```python
from build123d import *

# Parameters (mm, degrees)
TD_SKETCH_R                             = 0.79248
TL_FEATURE_DEPTH                        = 21.0312
TDF_STD_SKETCH_W                        = 2.09296
TDF_STD_SKETCH_H                        = 2.09296
TDF_STD_FEATURE_DEPTH                   = 22.061040395
ISA_20_STD_FEATURE_DEPTH                = 22.061040395
ISA_20_STD_FEATURE_DEPTH_BACK           = 22.061040395
F_10BA_STD_FEATURE_DEPTH                = 22.061040395
F_10BA_STD_FEATURE_DEPTH_BACK           = 22.061040395
FRO_STD_FEATURE_DEPTH                   = 22.061040395
FRO_STD_FEATURE_DEPTH_BACK              = 22.061040395
C_STD_FEATURE_DEPTH                     = 22.061040395
C_STD_FEATURE_DEPTH_BACK                = 22.061040395
ERW_STD_FEATURE_DEPTH                   = 0.028575
H_STD_FEATURE_REACH                     = 22.881
H_STD_SKETCH_R                          = 0.01905
H_STD_SKETCH_3_R                        = 0.01905
FUNNEL_FINAL_DIAMETRE_STD_FEATURE_DEPTH = 2.499995
FUNNEL_FINAL_DIAMETRE_STD_FEATURE_DRAFT = -22.5
ROUND_BR_STD_FEATURE_START              = -1
ROUND_BR_STD_FEATURE_DEPTH              = 1.020088772


with BuildPart() as part:
    # TD_sketch → TL_feature (new body)
    with BuildSketch(Plane(origin=(0, 0, 0), x_dir=(1, 0, 0), z_dir=(0, 1, 0))):
        with Locations(Location((0, 0, 0), (0, 0, 270))):
            Circle(TD_SKETCH_R)
    extrude(amount=TL_FEATURE_DEPTH)

    # TDF_STD_sketch → TDF_STD_feature (cut, through all)
    with BuildSketch(Plane(origin=(0, 0, 0), x_dir=(1, 0, 0), z_dir=(0, 1, 0))):
        with Locations((-1.4224, 0)):
            Rectangle(TDF_STD_SKETCH_W, TDF_STD_SKETCH_H)
    extrude(amount=TDF_STD_FEATURE_DEPTH, mode=Mode.SUBTRACT)

    # ISA_20_STD_sketch → ISA_20_STD_feature (cut, two sides: drawn at the far end of the back side and taken through both)
    with BuildSketch(Plane(origin=(0, 0, 0), x_dir=(0, 0, -1), z_dir=(1, 0, 0)).offset(-ISA_20_STD_FEATURE_DEPTH_BACK)):
        Polygon((-12.952451681, 73.255332957), (-3.743927997, 21.0312), (-0.03556, 0), (0.03556, 0), (3.743927997, 21.0312), (12.952451681, 73.255332957), (12.952451681, -32.804215817), (-12.952451681, -32.804215817), align=None)
    extrude(amount=ISA_20_STD_FEATURE_DEPTH + ISA_20_STD_FEATURE_DEPTH_BACK, mode=Mode.SUBTRACT)

    # 10BA_STD_sketch → 10BA_STD_feature (cut, two sides: drawn at the far end of the back side and taken through both)
    with BuildSketch(Plane.XY.offset(-F_10BA_STD_FEATURE_DEPTH_BACK)):
        Polygon((-53.226091717, 0), (-0.37592, 0), (-0.28702, 0), (0.014453164, 0.053157853), (3.713447997, 21.0312), (12.890784005, 73.078458855), (91.272293615, 2.163710365), (25.155417893, -70.914748491), align=None)
    extrude(amount=F_10BA_STD_FEATURE_DEPTH + F_10BA_STD_FEATURE_DEPTH_BACK, mode=Mode.SUBTRACT)

    # FRO_STD_sketch → FRO_STD_feature (cut, two sides: drawn at the far end of the back side and taken through both)
    with BuildSketch(Plane.XY.offset(-FRO_STD_FEATURE_DEPTH_BACK)):
        with BuildLine():
            Line((-0.37592, 52.147609748), (-0.37592, 0.02286))
            ThreePointArc((-0.37592, 0.02286), (-0.369224461, 0.006695539), (-0.35306, 0))
            Line((-0.35306, 0), (51.771689748, 0))
            Line((51.771689748, 0), (-21.943838281, -73.715528029))
            Line((-21.943838281, -73.715528029), (-74.091448029, -21.567918281))
            Line((-74.091448029, -21.567918281), (-0.37592, 52.147609748))
        make_face()
    extrude(amount=FRO_STD_FEATURE_DEPTH + FRO_STD_FEATURE_DEPTH_BACK, mode=Mode.SUBTRACT)

    # C_STD_sketch → C_STD_feature (cut, two sides: drawn at the far end of the back side and taken through both)
    with BuildSketch(Plane(origin=(0, 0, 0), x_dir=(0, 0, -1), z_dir=(1, 0, 0)).offset(-C_STD_FEATURE_DEPTH_BACK)):
        with BuildLine():
            Line((-50.946547499, -11.043402092), (-0.035537314, 0))
            ThreePointArc((-0.035537314, 0), (0, 0.00381), (0.035537314, 0))
            Line((0.035537314, 0), (50.946547499, -11.043402092))
            Line((50.946547499, -11.043402092), (50.946547499, -115.233376423))
            Line((50.946547499, -115.233376423), (-50.946547499, -115.233376423))
            Line((-50.946547499, -115.233376423), (-50.946547499, -11.043402092))
        make_face()
    extrude(amount=C_STD_FEATURE_DEPTH + C_STD_FEATURE_DEPTH_BACK, mode=Mode.SUBTRACT)


with BuildPart() as body_2:
    # ERW_STD_sketch → ERW_STD_feature (new, symmetric)
    with BuildSketch(Plane.XY):
        Polygon((-0.127, 0.09652), (-0.127, 0), (-0.3175, 0), (-0.261774152, 0.09652), align=None)
    extrude(amount=ERW_STD_FEATURE_DEPTH, both=True)

    # H_STD_sketch → H_STD_feature (add, up to next)
    with BuildSketch(Plane(origin=(0.01693898, 0.179623209, 0), x_dir=(0, 0, -1), z_dir=(0.8660254037844415, 0.4999999999999953, 0)), mode=Mode.PRIVATE) as h_std_feature_sk1:
        with Locations(Location((0, 0, 0), (0, 0, 90))):
            Circle(H_STD_SKETCH_R)
    h_std_feature_tool1 = extrude(h_std_feature_sk1.sketch, amount=-H_STD_FEATURE_REACH, mode=Mode.PRIVATE) - body_2.part
    add(h_std_feature_tool1.solids().sort_by_distance((0.016939, 0.179623, 0))[0])


with BuildPart() as funnel_final_diametre_std_feature_tool:
    # H_STD_sketch<3> → funnel_final_diametre_STD_feature (with draft: the straight prism first)
    with BuildSketch(Plane(origin=(0.01693898, 0.179623209, 0), x_dir=(0, 0, -1), z_dir=(0.8660254037844415, 0.4999999999999953, 0))):
        with Locations(Location((0, 0, 0), (0, 0, 90))):
            Circle(H_STD_SKETCH_3_R)
    extrude(amount=FUNNEL_FINAL_DIAMETRE_STD_FEATURE_DEPTH)
    # funnel_final_diametre_STD_feature: the draft: its side faces are tilted about the plane it starts from
    funnel_final_diametre_std_feature_sides = [funnel_final_diametre_std_feature_tool.faces().sort_by_distance(p)[0] for p in [
        (1.10899357, 0.788124175, 0),
    ]]
    draft(funnel_final_diametre_std_feature_sides, Plane(origin=(0.01693898, 0.179623209, 0), x_dir=(0, 0, -1), z_dir=(0.8660254037844415, 0.4999999999999953, 0)), FUNNEL_FINAL_DIAMETRE_STD_FEATURE_DRAFT)


with BuildPart() as body_2_1:
    add(body_2.part)

    # funnel_final_diametre_STD_feature: add funnel_final_diametre_std_feature_tool
    add(funnel_final_diametre_std_feature_tool.part)

    # ROUND_BR_STD_feature: read off the stored shape, not the designer's step
    # ROUND_BR_STD_feature outline → ROUND_BR_STD_feature (cut)
    with BuildSketch(Plane(origin=(0, 0, 0), x_dir=(0.8660254037844362, -0.5000000000000042, 0), z_dir=(0.5000000000000042, 0.8660254037844363, 0)).offset(ROUND_BR_STD_FEATURE_START)):
        with BuildLine():
            Line((-0.274963066, -0.028575), (-0.246388066, -0.028575))
            ThreePointArc((-0.246388066, -0.028575), (-0.266593642, -0.020205576), (-0.274963066, 0))
            Line((-0.274963066, 0), (-0.274963066, -0.028575))
        make_face()
        with BuildLine():
            Line((-0.274963066, 0.028575), (-0.274963066, 0))
            ThreePointArc((-0.274963066, 0), (-0.266593642, 0.020205576), (-0.246388066, 0.028575))
            Line((-0.246388066, 0.028575), (-0.274963066, 0.028575))
        make_face()
    extrude(amount=ROUND_BR_STD_FEATURE_DEPTH, mode=Mode.SUBTRACT)


with BuildPart() as part_1:
    add(part.part)

    # COMBINE_STD_feature: cut body 2
    add(body_2_1.part, mode=Mode.SUBTRACT)


solid = part_1.part
```
Verification items for the finished model (mm, model axes). Round coordinates to 2 decimals unless told otherwise and drop trailing zeros. Order: outer loops, then holes, each group sorted by start corner. A loop starts at its lowest first (then second) coordinate and runs counter-clockwise, first axis right, second up. Notation, with made-up numbers: (30.5, -39.5) -> (62.5, -39.5) arc R19 ccw to (62.5, -11.5) -> close; hole circle Ø5 at (22, 69.25). An arc over 180 degrees is marked (long way). Put each result on its own line as item: value. Start each with the question number.
(1) Section check C-C (z = -0.3). Enter the section's corners in (x, y), then the cut area to 3 significant figures.
(2) Section check B-B (y = 18.5). Enter the section's corners in (x, z).
(3) Material ranges on line 1 along X through (y, z) = (18.75, -0.05); line 2 along Z through (x, y) = (0.25, 6.5); line 3 along X through (y, z) = (11.5, 0.4), recorded low to high.
(4) Section check D-D (y = 1.5). Enter the section's corners in (x, z).
(5) Section check A-A (x = 0.25). Enter the section's corners in (y, z).
Completed:
1. outline: (-0.38, 1.5) -> (0.27, 1.5) -> (0.73, 4.13) -> (0.73, 21.03) -> (-0.38, 21.03) -> close
1. area: 21.1 mm2
2. outline: (-0.38, -0.7) arc R0.79 ccw (long way) to (-0.38, 0.7) -> close
3. line 1: x = -0.38 to 0.79
3. line 2: z = -0.75 to 0.75
3. line 3: x = -0.38 to 0.68
4. outline: (-0.38, -0.3) -> (0.27, -0.3) -> (0.27, 0.3) -> (-0.38, 0.3) -> close
5. outline: (1.39, -0.28) -> (4.06, -0.75) -> (21.03, -0.75) -> (21.03, 0.75) -> (4.06, 0.75) -> (1.39, 0.28) -> close
